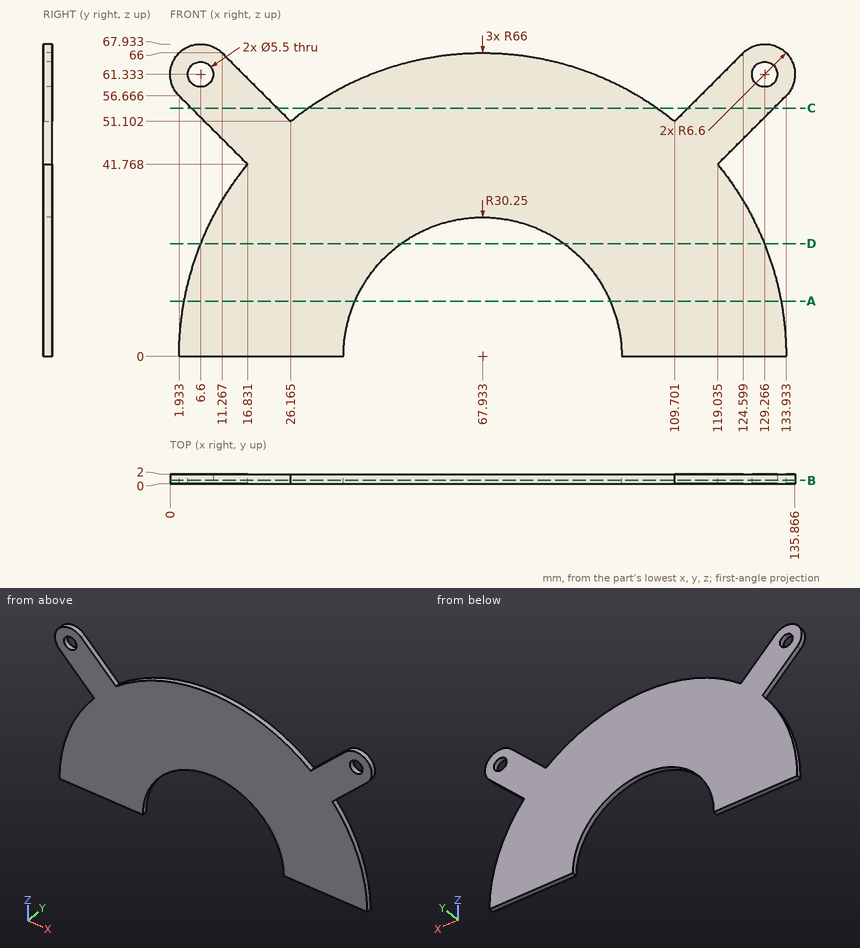
Input: dimensioned drawing with shaded views. Units: mm. Origin: part minimum x, y, z. Give positions to 0.01 mm unless a question says otherwise; leave off trailing zeros. Loops run counter-clockwise (first coordinate to the right, second up) from the corner with the lowest first, then second, coordinate; pieces in that order, holes last. Notation, with made-up numbers: (-4, 68) -> (9, 68) arc R23 ccw to (9, 93) -> close; hole circle Ø5 at (-26.75, 23.5). An arc over 180 degrees is marked (long way). Use a Markdown table: item, result. Add a question column.
1) Section query C-C, the plane z = 54. Return the cut outline in (x, y).
2) Section query B-B, the plane y = 0.7. Count the separate pieces of the cut face and the enclosed holes in it.
3) Section query D-D, the plane z = 24.5. Return the cut outline in (x, y).
4) First-contact query: pin 1 (1 mm diameter, centred on y = 1, z = 20, fed in from -X). Flat tip, straight axial feed; report the tip coordinate or a pass-through.
5) Section query A-A, the plane z = 12. Return the cut outline in (x, y) (1 decimal).
6) Line query: line 1 along Z through (x, y) = (127, 1.1) (1 decimal); line 2 along Z through (x, y) = (8.5, 1.1) (1 decimal); line 3 along X through (y, z) = (1.7, 54) (1 decimal). Output: solid intervals per line, ascending. Write a range as [from, to].
Numbers:
| question | item | result |
|---|---|---|
| 1 | outline | (4.6, 0) -> (23.27, 0) -> (23.27, 2) -> (4.6, 2) -> close; (29.99, 0) -> (105.88, 0) -> (105.88, 2) -> (29.99, 2) -> close; (112.6, 0) -> (131.27, 0) -> (131.27, 2) -> (112.6, 2) -> close |
| 2 | separate pieces | 1 |
| 2 | enclosed holes | 2 |
| 3 | outline | (6.65, 0) -> (50.19, 0) -> (50.19, 2) -> (6.65, 2) -> close; (85.68, 0) -> (129.22, 0) -> (129.22, 2) -> (85.68, 2) -> close |
| 4 | pin 1 | stops at x = 4.88 |
| 5 | outline | (3, 0) -> (40.2, 0) -> (40.2, 2) -> (3, 2) -> close; (95.7, 0) -> (132.8, 0) -> (132.8, 2) -> (95.7, 2) -> close |
| 6 | line 1 | z = [0, 29.4], [49.7, 59.8], [62.9, 67.5] |
| 6 | line 2 | z = [0, 28.7], [50.1, 59.3], [63.3, 67.7] |
| 6 | line 3 | x = [4.6, 23.3], [30, 105.9], [112.6, 131.3] |
